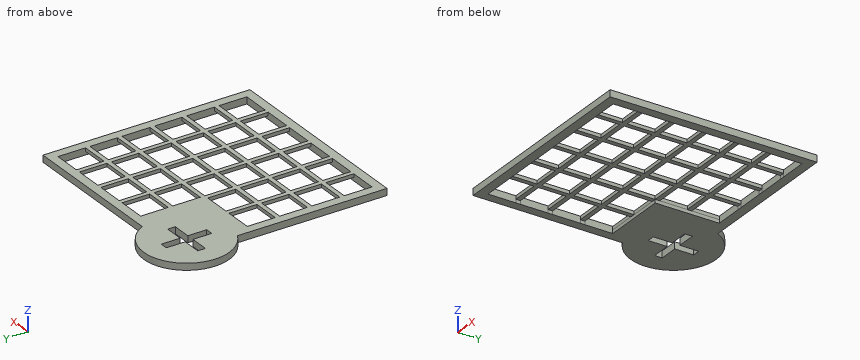
```python
from build123d import *

# Parameters (mm, degrees)
PAD039_DEPTH    = 3
SKETCH067_W     = 12.2279220614
SKETCH067_H     = 12.4149860738
SKETCH067_H_2   = 12.2902767322
SKETCH067_H_3   = 12.352631403
SKETCH067_W_2   = 12.4149860738
SKETCH067_W_3   = 12.2902767322
SKETCH067_W_4   = 12.352631403
SKETCH067_H_4   = 12.2279220614
POCKET027_DEPTH = 3.001
POCKET028_DEPTH = 1.5


with BuildPart() as part:
    # Sketch066 (on Face3 of Binder013) → Pad039 (new body)
    with BuildSketch(Plane.XY.offset(18.2)):
        with BuildLine():
            ThreePointArc((-66.6105256119, 92.0663697346), (-97.0746391493, 97.0746391493), (-92.0663697346, 66.6105256119))
            Line((-92.0663697346, 66.6105256119), (-92.0663697346, 0.2))
            Line((-92.0663697346, 0.2), (-0.2, 0.2))
            Line((-0.2, 92.0663697346), (-0.2, 0.2))
            Line((-66.6105256119, 92.0663697346), (-0.2, 92.0663697346))
        make_face()
    extrude(amount=PAD039_DEPTH)

    # Sketch067 (on Face7 of Pad039) → Pocket027 (cut, through all)
    with BuildSketch(Plane.XY.offset(21.2)):
        Polygon((-93.7396103068, 85.3396103068), (-85.3396103068, 85.3396103068), (-85.3396103068, 93.7396103068), (-81.9396103068, 93.7396103068), (-81.9396103068, 85.3396103068), (-73.5396103068, 85.3396103068), (-73.5396103068, 81.9396103068), (-81.9396103068, 81.9396103068), (-81.9396103068, 73.5396103068), (-85.3396103068, 73.5396103068), (-85.3396103068, 81.9396103068), (-93.7396103068, 81.9396103068), align=None)
        with Locations((-81.9524087039, 53.403032575)):
            Rectangle(SKETCH067_W, SKETCH067_H)
        with Locations((-67.7244866426, 53.403032575)):
            Rectangle(SKETCH067_W, SKETCH067_H)
        with Locations((-81.9524087039, 39.050401172)):
            Rectangle(SKETCH067_W, SKETCH067_H_2)
        with Locations((-67.7244866426, 39.050401172)):
            Rectangle(SKETCH067_W, SKETCH067_H_2)
        with Locations((-81.9524087039, 24.7289471045)):
            Rectangle(SKETCH067_W, SKETCH067_H_3)
        with Locations((-67.7244866426, 24.7289471045)):
            Rectangle(SKETCH067_W, SKETCH067_H_3)
        with Locations((-81.9524087039, 10.3763157015)):
            Rectangle(SKETCH067_W, SKETCH067_H_3)
        with Locations((-67.7244866426, 10.3763157015)):
            Rectangle(SKETCH067_W, SKETCH067_H_3)
        with Locations((-53.403032575, 10.3763157015)):
            Rectangle(SKETCH067_W_2, SKETCH067_H_3)
        with Locations((-39.050401172, 10.3763157015)):
            Rectangle(SKETCH067_W_3, SKETCH067_H_3)
        with Locations((-24.7289471045, 10.3763157015)):
            Rectangle(SKETCH067_W_4, SKETCH067_H_3)
        with Locations((-10.3763157015, 10.3763157015)):
            Rectangle(SKETCH067_W_4, SKETCH067_H_3)
        with Locations((-10.3763157015, 24.7601244399)):
            Rectangle(SKETCH067_W_4, SKETCH067_H_2)
        with Locations((-24.7289471045, 24.7601244399)):
            Rectangle(SKETCH067_W_4, SKETCH067_H_2)
        with Locations((-39.050401172, 24.7601244399)):
            Rectangle(SKETCH067_W_3, SKETCH067_H_2)
        with Locations((-53.403032575, 24.7289471045)):
            Rectangle(SKETCH067_W_2, SKETCH067_H_3)
        with Locations((-53.403032575, 39.050401172)):
            Rectangle(SKETCH067_W_2, SKETCH067_H_2)
        with Locations((-39.050401172, 39.050401172)):
            Rectangle(SKETCH067_W_3, SKETCH067_H_2)
        with Locations((-24.7289471045, 39.050401172)):
            Rectangle(SKETCH067_W_4, SKETCH067_H_2)
        with Locations((-10.3763157015, 39.050401172)):
            Rectangle(SKETCH067_W_4, SKETCH067_H_2)
        with Locations((-10.3763157015, 53.403032575)):
            Rectangle(SKETCH067_W_4, SKETCH067_H)
        with Locations((-24.7289471045, 53.403032575)):
            Rectangle(SKETCH067_W_4, SKETCH067_H)
        with Locations((-39.050401172, 53.403032575)):
            Rectangle(SKETCH067_W_3, SKETCH067_H)
        with Locations((-53.403032575, 53.403032575)):
            Rectangle(SKETCH067_W_2, SKETCH067_H)
        with Locations((-53.403032575, 67.7244866426)):
            Rectangle(SKETCH067_W_2, SKETCH067_H_4)
        with Locations((-39.050401172, 67.7244866426)):
            Rectangle(SKETCH067_W_3, SKETCH067_H_4)
        with Locations((-24.7289471045, 67.7244866426)):
            Rectangle(SKETCH067_W_4, SKETCH067_H_4)
        with Locations((-10.3763157015, 67.7244866426)):
            Rectangle(SKETCH067_W_4, SKETCH067_H_4)
        with Locations((-10.3763157015, 81.9524087039)):
            Rectangle(SKETCH067_W_4, SKETCH067_H_4)
        with Locations((-24.7289471045, 81.9524087039)):
            Rectangle(SKETCH067_W_4, SKETCH067_H_4)
        with Locations((-39.050401172, 81.9524087039)):
            Rectangle(SKETCH067_W_3, SKETCH067_H_4)
        with Locations((-53.403032575, 81.9524087039)):
            Rectangle(SKETCH067_W_2, SKETCH067_H_4)
    extrude(amount=-POCKET027_DEPTH, mode=Mode.SUBTRACT)

    # Sketch068 (on Face4 of Pocket027) → Pocket028 (cut)
    with BuildSketch(Plane(origin=(0, 0, 18.2), x_dir=(1, 0, 0), z_dir=(0, 0, -1))):
        Polygon((-88.06637, -4.2), (-4.2, -4.2), (-4.2, -88.06637), (-59.610526, -88.06637), (-59.610526, -59.610526), (-88.06637, -59.610526), align=None)
    extrude(amount=-POCKET028_DEPTH, mode=Mode.SUBTRACT)


solid = part.part
```
Build history of the part. All positions in model axes, mm. Round coordinates to 2 decimals unless told otherwise and drop trailing zeros. Write each loop counter-clockwise with the first axis right and the second up, starting at its lowest first coordinate (ties: lowest second). Pieces come first, ordered by that corner, then holes.
1) Band-saw the part on C-C, the plane x = -22. List the corners of the cut face in (y, z).
2) Drill centre lines: probe 1 along Y at (x, z) = (-62.5, 20.5); probe 2 along Y at (x, z) = (-11.5, 18.5); probe 3 along X at (y, z) = (85, 19.9). Where is each one in solid material? Low to high.
3) Band-saw the part on A-A, the plane y = 54.5. List the corners of the cut face in (x, z), and give its area (3 significant figures).
4) Band-saw the part on B-B, the plane z = 18.9. List the corners of the cut face in (x, y), and give its area (3 significant figures).
5) Pin check, flat tips, straight feed: pin 1 (0.8 mm diameter, centred on x = -41, z = 20.5, fed in from +Y); pin 2 (0.8 mm diameter, centred on y = 50.5, z = 20.5, fed in from -X); pin 3 (1.5 mm diameter, centred on x = -89.5, z = 20, fed in from +Y). Stop position of each tip, or through.
6) Band-saw the part on D-D, the plane y = 77. List the corners of the cut face in (x, z), and give its area (3 significant figures).
Ans:
1. outline: (0.2, 18.2) - (4.2, 18.2) - (4.2, 21.2) - (0.2, 21.2) - close; (16.55, 19.7) - (18.61, 19.7) - (18.61, 21.2) - (16.55, 21.2) - close; (30.91, 19.7) - (32.91, 19.7) - (32.91, 21.2) - (30.91, 21.2) - close; (45.2, 19.7) - (47.2, 19.7) - (47.2, 21.2) - (45.2, 21.2) - close; (59.61, 19.7) - (61.61, 19.7) - (61.61, 21.2) - (59.61, 21.2) - close; (73.84, 19.7) - (75.84, 19.7) - (75.84, 21.2) - (73.84, 21.2) - close; (88.07, 18.2) - (92.07, 18.2) - (92.07, 21.2) - (88.07, 21.2) - close
2. probe 1: y = 0.2 to 4.2, 16.55 to 18.55, 30.91 to 32.91, 45.2 to 47.2, 59.61 to 92.07
2. probe 2: y = 0.2 to 4.2, 88.07 to 92.07
2. probe 3: x = -102.59 to -93.74, -73.54 to -59.61, -47.2 to -45.2, -32.91 to -30.91, -18.55 to -16.55, -4.2 to -0.2
3. outline: (-92.07, 18.2) - (-88.07, 18.2) - (-88.07, 21.2) - (-92.07, 21.2) - close; (-75.84, 19.7) - (-73.84, 19.7) - (-73.84, 21.2) - (-75.84, 21.2) - close; (-61.61, 19.7) - (-59.61, 19.7) - (-59.61, 21.2) - (-61.61, 21.2) - close; (-47.2, 19.7) - (-45.2, 19.7) - (-45.2, 21.2) - (-47.2, 21.2) - close; (-32.91, 19.7) - (-30.91, 19.7) - (-30.91, 21.2) - (-32.91, 21.2) - close; (-18.55, 19.7) - (-16.55, 19.7) - (-16.55, 21.2) - (-18.55, 21.2) - close; (-4.2, 18.2) - (-0.2, 18.2) - (-0.2, 21.2) - (-4.2, 21.2) - close
3. area: 39.0 mm2
4. outline: (-92.07, 0.2) - (-0.2, 0.2) - (-0.2, 92.07) - (-66.61, 92.07) arc R19 ccw (long way) to (-92.07, 66.61) - close; hole (-93.74, 81.94) - (-85.34, 81.94) - (-85.34, 73.54) - (-81.94, 73.54) - (-81.94, 81.94) - (-73.54, 81.94) - (-73.54, 85.34) - (-81.94, 85.34) - (-81.94, 93.74) - (-85.34, 93.74) - (-85.34, 85.34) - (-93.74, 85.34) - close; hole (-88.07, 4.2) - (-4.2, 4.2) - (-4.2, 88.07) - (-59.61, 88.07) - (-59.61, 59.61) - (-88.07, 59.61) - close
4. area: 2,560 mm2
5. pin 1: stops at y = 92.07
5. pin 2: stops at x = -92.07
5. pin 3: stops at y = 101.94
6. outline: (-101.44, 18.2) - (-85.34, 18.2) - (-85.34, 21.2) - (-101.44, 21.2) - close; (-81.94, 18.2) - (-59.61, 18.2) - (-59.61, 21.2) - (-81.94, 21.2) - close; (-47.2, 19.7) - (-45.2, 19.7) - (-45.2, 21.2) - (-47.2, 21.2) - close; (-32.91, 19.7) - (-30.91, 19.7) - (-30.91, 21.2) - (-32.91, 21.2) - close; (-18.55, 19.7) - (-16.55, 19.7) - (-16.55, 21.2) - (-18.55, 21.2) - close; (-4.2, 18.2) - (-0.2, 18.2) - (-0.2, 21.2) - (-4.2, 21.2) - close
6. area: 136 mm2
